from build123d import *

# Parameters (mm, degrees)
F1_DEPTH    = 2.6
F2_T1_DEPTH = 15.1
F2_T3_DEPTH = 15.009673646
F3_R        = 4.32
F4_DEPTH    = 1.66
F5_R        = 3.375
F6_DEPTH    = 7.3
F7_R        = 1


# Not quite as in the source:
# - a fillet or chamfer that OpenCascade refuses, or shapes differently, is made with other operations: its cross-section is extruded or revolved along the edge and cut away or added


with BuildPart() as f1:
    # F0 (on Top) → F1 (new body)
    with BuildSketch(Plane.XY):
        Polygon((0, 12.5), (0, 0), (45.4, 0), (45.4, 31.6), (0, 31.6), (0, 19.1), (2.2, 19.1), (2.2, 12.5), align=None)
    extrude(amount=F1_DEPTH)

    # F2: fillet of radius 2.5 on 6 edges, made by hand

    # F2_s2 → F2_t1 (cut)
    with BuildSketch(Plane.XY.offset(-6.25)):
        with BuildLine():
            ThreePointArc((45.4, 29.1), (44.667766953, 30.867766953), (42.9, 31.6))
            Line((42.9, 31.6), (45.4, 31.6))
            Line((45.4, 31.6), (45.4, 29.1))
        make_face()
        with BuildLine():
            ThreePointArc((2.5, 31.6), (0.732233047, 30.867766953), (0, 29.1))
            Line((0, 29.1), (0, 31.6))
            Line((0, 31.6), (2.5, 31.6))
        make_face()
        with BuildLine():
            ThreePointArc((42.9, 0), (44.667766953, 0.732233047), (45.4, 2.5))
            Line((45.4, 2.5), (45.4, 0))
            Line((45.4, 0), (42.9, 0))
        make_face()
        with BuildLine():
            ThreePointArc((0, 2.5), (0.732233047, 0.732233047), (2.5, 0))
            Line((2.5, 0), (0, 0))
            Line((0, 0), (0, 2.5))
        make_face()
    extrude(amount=F2_T1_DEPTH, mode=Mode.SUBTRACT)

    # F2_s4 → F2_t3 (cut)
    with BuildSketch(Plane.XY.offset(-6.204836823)):
        with BuildLine():
            ThreePointArc((0, 21.5819347292), (0.6291713066, 19.923622334), (2.2, 19.1))
            Line((2.2, 19.1), (0, 19.1))
            Line((0, 19.1), (0, 21.5819347292))
        make_face()
        with BuildLine():
            ThreePointArc((0, 10.0180652708), (0.6291713066, 11.676377666), (2.2, 12.5))
            Line((2.2, 12.5), (0, 12.5))
            Line((0, 12.5), (0, 10.0180652708))
        make_face()
    extrude(amount=F2_T3_DEPTH, mode=Mode.SUBTRACT)

    # F3 (on face) → F4 (join)
    with BuildSketch(Plane.XY.offset(2.6)):
        with Locations((23.49, 16.68)):
            Circle(F3_R)
    extrude(amount=F4_DEPTH)

    # F5 (on face) → F6 (join)
    with BuildSketch(Plane.XY.offset(4.26)):
        with Locations((23.49, 16.68)):
            Circle(F5_R)
    extrude(amount=F6_DEPTH)

    # F7
    f7_edges = [f1.edges().sort_by_distance(p)[0] for p in [
        (20.115, 16.68, 11.56),
    ]]
    fillet(f7_edges, radius=F7_R)


solid = f1.part
Geometry check sheet. Reference: the model listing, model coordinates, mm. A direction names the side the tool comes from. Give positions to 0.01 mm unless a question says otherwise; leave off trailing zeros. Write each loop counter-clockwise with the first axis right and the second up, starting at its lowest first coordinate (ties: lowest second). Pieces come first, ordered by that corner, then holes.
1) Cross-section at B-B (x = 23.49). Record the boundary of the cut face in (y, z) (3 decimals), plus the area to 3 significant figures.
Values follow:
outline: (0, 0) - (31.6, 0) - (31.6, 2.6) - (21, 2.6) - (21, 4.26) - (20.055, 4.26) - (20.055, 10.56) arc R1 ccw to (19.055, 11.56) - (14.305, 11.56) arc R1 ccw to (13.305, 10.56) - (13.305, 4.26) - (12.36, 4.26) - (12.36, 2.6) - (0, 2.6) - close
area: 145 mm2
2) Cross-section at A-A (y = 16.68). Record the boundary of the cut face in (x, z) (3 decimals).
Values follow:
outline: (2.2, 0) - (45.4, 0) - (45.4, 2.6) - (27.81, 2.6) - (27.81, 4.26) - (26.865, 4.26) - (26.865, 10.56) arc R1 ccw to (25.865, 11.56) - (21.115, 11.56) arc R1 ccw to (20.115, 10.56) - (20.115, 4.26) - (19.17, 4.26) - (19.17, 2.6) - (2.2, 2.6) - close
3) Thickness scan on line 1 (Z direction, x = 19.5, y = 3.5); line 2 (X direction, y = 16, z = 0.75); line 3 (Y direction, x = 20.5, z = 10.5). Record the ranges inside material, lowest first.
Values follow:
line 1: z = 0 to 2.6
line 2: x = 2.2 to 45.4
line 3: y = 15.11 to 18.25
4) Cross-section at D-D (z = 3.25). Record the boundary of the cut face in (x, y), plus the area to 3 significant figures.
Values follow:
outline: circle Ø8.64 at (23.49, 16.68)
area: 58.6 mm2
5) Release check for a two-part mould opening along Y. For faces 4 (the face through (22, 16, 0)), 5 (the face through (0.713, 0.752, 1.282)), 6 (the face through (2.2, 16, 1)) record: released by +Y, released by -Y, zero draft, split by the parting line, or undercut.
Values follow:
face 4: zero draft
face 5: released by -Y
face 6: undercut
6) Cross-section at C-C (z = 10). Record the boundary of the cut face in (x, y) (3 decimals), plus the area to 3 significant figures.
Values follow:
outline: circle Ø6.75 at (23.49, 16.68)
area: 35.8 mm2
7) Go/stop test with flat-tipped pins: pin 1 Ø0.8 at (y, z) = (15.5, 1) entering from -X; pin 2 Ø1.5 at (y, z) = (13, 9) entering from +X (3 decimals); pin 3 Ø5 at (x, y) = (38.5, 12.5) entering from +Z. Record where each tip stops, or that it passes through.
Values follow:
pin 1: stops at x = 2.2
pin 2: stops at x = 25.165
pin 3: stops at z = 2.6
8) Set-up check for faces 1 (the face through (0.612, 19.943, 1.282)), 2 (the face through (20.062, 14.051, 3.418)), 3 (the face through (44.648, 0.713, 1.282)): record each of +Z, -Z, +X, -X, +Y, -Y from which the full face is reachable in a straight line by a thin tool's end or side.
Values follow:
face 1: +Z, -Z, -X
face 2: +Z
face 3: +Z, -Z, +X, -Y
